from build123d import *

# Parameters (mm, degrees)
F2_R     = 5.08
F4_D     = 12.7
F4_DEPTH = 90.273154499


with BuildPart() as f1:
    # F0 (on Front) → F1 (revolve)
    with BuildSketch(Plane.XZ):
        with BuildLine():
            ThreePointArc((-91.9005685167, 39.3456475336), (-49.9844837763, 10.2500476162), (0, 0))
            Line((0, 0), (0, 127))
            Line((0, 127), (-25.4, 127))
            Line((-25.4, 127), (-91.9005685167, 39.3456475336))
        make_face()
    revolve(axis=Axis((0, 0, 63.5), (0, 0, 1)))

    # F2
    f2_edges = [f1.edges().sort_by_distance(p)[0] for p in [
        (91.900569, 0, 39.345648),
    ]]
    fillet(f2_edges, radius=F2_R)

    # F4 (through all, one way)
    with BuildSketch(Plane.XZ):
        with Locations((0, 112.6990020275)):
            Circle(F4_D / 2)
    extrude(amount=-F4_DEPTH, mode=Mode.SUBTRACT)


solid = f1.part
For this review, take the finished solid that the model builds, in its own axes (mm). A direction names the side the tool comes from. Coordinates: 2 decimals unless noted, no trailing zeros. Loops run counter-clockwise (first coordinate to the right, second up) from the corner with the lowest first, then second, coordinate; pieces in that order, holes last. Notation, with made-up numbers: (9.5, 69) - (52.5, 69) arc R17 ccw to (52.5, 84) - close; hole circle Ø7 at (-14.5, 75). An arc over 180 degrees is marked (long way). Use a Markdown table: item, result. Add a question column.
Item 1: We need section A-A (z = 109). Give the boundary of the cut face in (x, y), and give its area (3 significant figures).
Item 2: For line 1 (Y direction, x = -13.5, z = 40); line 2 (Z direction, x = 0, y = 24); line 3 (Z direction, x = 0, y = 14), list the stretches that pass through material, from the lowest coordinate up.
Item 3: Tool access review of faces 1 (the face through (0, 0, 127)), 2 (the face through (-1.38, 20.25, 106.5)): name each direction out of +Z, -Z, +X, -X, +Y, -Y from which nothing blocks a thin tool from reaching the whole face with its end or side.
Item 4: We need section C-C (z = 31.5). Give the boundary of the cut face in (x, y), and give its area (3 significant figures).
Item 5: Insertion check: pin 1 Ø2 at (x, y) = (6, -55) entering from +Z; pin 2 Ø5 at (x, z) = (45, 40.5) entering from -Y; pin 3 Ø4 at (x, y) = (19.5, -60) entering from -Z. Each pin has a flat end and moves straight along its axis. Give the tip position at first contact, or say it passes through.
Item 6: We need section B-B (z = 59.5). Give the boundary of the cut face in (x, y).
Item 7: Mouldability with a two-part tool opening along Z and no side actions: class faces 3 (the face through (0, 0, 113)), 4 (the face through (-34.8, -10.96, 112.39)) as pulls with the +Z half, pulls with the -Z half, needs draft (parallel to the pull), parting line crosses it, or undercut.
Results list:
| question | item | result |
|---|---|---|
| 1 | outline | (-5.16, 0) - (-5.16, 38.71) arc R39.06 ccw (long way) to (5.16, 38.71) - (5.16, 0) - close |
| 1 | area | 4,390 mm^2 |
| 2 | line 1 | y = -89.25 to 89.25 |
| 2 | line 2 | z = 2.29 to 106.35, 119.05 to 127 |
| 2 | line 3 | z = 0.77 to 106.35, 119.05 to 127 |
| 3 | face 1 | +Z, +X, -X, +Y, -Y |
| 3 | face 2 | +Y |
| 4 | outline | circle Ø167.44 at (0, 0) |
| 4 | area | 22,000 mm^2 |
| 5 | pin 1 | stops at z = 88.87 |
| 5 | pin 2 | stops at y = -79.61 |
| 5 | pin 3 | stops at z = 15.66 |
| 6 | outline | circle Ø153.22 at (0, 0) |
| 7 | face 3 | undercut |
| 7 | face 4 | pulls with the +Z half |
